Autodesk Fusion 360 part; units mm, degrees
sketch "Sketch1" plane through (0, 0, 0) normal (0, 0, 1) x (1, 0, 0)
  line L0 (89, 44) -> (69, 44)
  line L1 (43, -56) -> (63, -56)
  line L2 (-89, 24) -> (-69, 24)
  line L3 (-124, 33) -> (-124, 53)
  line L4 (-95, 36) -> (-95, 56)
  line L5 (174, 69) -> (-174, 69)
  line L6 (-174, -69) -> (174, -69)
  line L7 (170, 37) -> (150, 37)
  line L8 (150, 37) -> (150, -2)
  line L9 (-183, 60) -> (-183, -60)
  line L10 (-124, 53) -> (-144, 53)
  line L11 (115, 56) -> (95, 56)
  line L12 (-150, 37) -> (-170, 37)
  line L13 (-170, 37) -> (-170, 17)
  line L14 (-89, 44) -> (-89, 24)
  line L15 (-62, -36) -> (-62, -23)
  line L16 (-115, 36) -> (-95, 36)
  line L17 (-69, 24) -> (-69, 44)
  line L18 (-69, 44) -> (-89, 44)
  line L19 (-62, -23) -> (-82, -23)
  line L20 (124, 14) -> (144, 14)
  line L21 (-144, 33) -> (-124, 33)
  circle A0 centre (173, -59) radius 2.6
  line L22 (-10, -30) -> (10, -30)
  line L23 (82, -30) -> (101, -30)
  line L24 (-43, -56) -> (-43, -36)
  line L25 (-63, -43) -> (-63, -56)
  line L26 (-82, -43) -> (-63, -43)
  circle A1 centre (-173, -59) radius 2.6
  line L27 (-144, 53) -> (-144, 33)
  line L28 (-10, -10) -> (-10, -30)
  line L29 (-150, 17) -> (-150, 37)
  line L30 (-115, 56) -> (-115, 36)
  line L31 (-63, -56) -> (-43, -56)
  line L32 (-170, 17) -> (-150, 17)
  line L33 (82, 3) -> (62, 3)
  line L34 (115, 17) -> (115, 56)
  line L35 (43, -30) -> (62, -30)
  line L36 (170, -2) -> (170, 37)
  line L37 (95, 56) -> (95, 17)
  line L38 (63, -43) -> (82, -43)
  line L39 (89, 5) -> (89, 44)
  circle A2 centre (0, -59) radius 2.6
  line L40 (183, -60) -> (183, 60)
  circle A3 centre (-173, 59) radius 2.6
  line L41 (43, -36) -> (43, -56)
  line L42 (62, 3) -> (62, -10)
  line L43 (69, 44) -> (69, 5)
  line L44 (10, -10) -> (-10, -10)
  line L45 (43, -10) -> (43, -30)
  line L46 (101, -30) -> (101, -10)
  line L47 (144, 53) -> (124, 53)
  line L48 (62, -10) -> (43, -10)
  line L49 (82, -43) -> (82, -30)
  line L50 (-95, 56) -> (-115, 56)
  line L51 (-82, -23) -> (-82, -43)
  line L52 (124, 53) -> (124, 14)
  line L53 (150, -2) -> (170, -2)
  circle A4 centre (173, 59) radius 2.6
  line L54 (62, -30) -> (62, -36)
  line L55 (10, -30) -> (10, -10)
  line L56 (95, 17) -> (115, 17)
  line L57 (101, -10) -> (82, -10)
  line L58 (62, -36) -> (43, -36)
  line L59 (82, -10) -> (82, 3)
  line L60 (63, -56) -> (63, -43)
  line L61 (69, 5) -> (89, 5)
  line L62 (144, 14) -> (144, 53)
  line L63 (-43, -36) -> (-62, -36)
  arc A5 (-174, 69) -> (-183, 60) centre (-174, 60) ccw
  arc A6 (183, 60) -> (174, 69) centre (174, 60) ccw
  arc A7 (174, -69) -> (183, -60) centre (174, -60) ccw
  arc A8 (-183, -60) -> (-174, -69) centre (-174, -60) ccw
  circle A9 centre (33, 54) radius 3.5
  circle A10 centre (-33, 54) radius 3.5
  circle A11 centre (33, 20) radius 3.5
  circle A12 centre (-33, 20) radius 3.5
  circle A13 centre (53, 59) radius 2.6
  circle A14 centre (-53, 59) radius 2.6
  dimension "d1" = 9
  dimension "d2" = 7
  dimension "d3" = 7
  dimension "d4" = 7
  dimension "d5" = 7
  dimension "d8" = 5.2
  dimension "d9" = 5.2
extrude "Extrude1" add sketch "Sketch1" along normal blind 6
Input: part model. Units: mm. Frame: model coordinates. A direction names the side the tool comes from. Coordinates: 2 decimals unless noted, no trailing zeros. Loops run counter-clockwise (first coordinate to the right, second up) from the corner with the lowest first, then second, coordinate; pieces in that order, holes last. Notation, with made-up numbers: M 68.25,59.25 L 81.25,59.25 A29 cw 81.25,89.25 Z; hole C 84,65.25 d5. An arc over 180 degrees is marked long. Use a Markdown table: item, result. Add a question column.
1) Section C-C, the plane x = -159. Return the cut outline in (y, z), plus the area to 3 significant figures.
2) Draft query along X for faces 3 (the flat face through (183, -1, 3)), 4 (the flat face through (134, 53, 3)), 5 (the flat face through (-2, -69, 3)), 6 (the cylindrical face through (-33.46, 16.53, 2.96)). Return one class per face: +X half, -X half, draft (parallel to the pull), parting line (faces both ways), or undercut.
3) Section D-D, the plane z = 2.05. Give the number of separate pieces and of enclosed holes in the cut face, plus the area to 3 significant figures.
4) Line query: L1, parallel to X at y = -32.5, z = 0.85; L2, parallel to Y at x = 69.5, z = 1.25; L3, parallel to X at y = -19, z = 5.6. Output: solid intervals per line, ascending. Write a range as from..to.
5) Section A-A, the plane x = -33. Return the cut outline in (y, z), plus the area to 3 significant figures.
6) Section B-B, the plane y = -16. Return the cut outline in (x, z), plus the area to 3 significant figures.
7) Set-up query: faces 1 (the flat face through (69, 25, 3)), 2 (the flat face through (-3, 1, 0)). Return all of +Z, -Z, +X, -X, +Y, -Y with unobstructed straight access to the full face (end or side cutting, diameter ignored); none if empty.
Answer below:
| question | item | result |
|---|---|---|
| 1 | outline | M -69,0 L 17,0 L 17,6 L -69,6 Z; M 37,0 L 69,0 L 69,6 L 37,6 Z |
| 1 | area | 708 mm2 |
| 2 | face 3 | +X half |
| 2 | face 4 | undercut |
| 2 | face 5 | draft |
| 2 | face 6 | undercut |
| 3 | separate pieces | 1 |
| 3 | enclosed holes | 22 |
| 3 | area | 42,100 mm2 |
| 4 | L1 | -183..-82, -62..62, 82..183 |
| 4 | L2 | -69..-43, 3..5, 44..69 |
| 4 | L3 | -183..-10, 10..43, 101..183 |
| 5 | outline | M -69,0 L 16.5,0 L 16.5,6 L -69,6 Z; M 23.5,0 L 50.5,0 L 50.5,6 L 23.5,6 Z; M 57.5,0 L 69,0 L 69,6 L 57.5,6 Z |
| 5 | area | 744 mm2 |
| 6 | outline | M -183,0 L -10,0 L -10,6 L -183,6 Z; M 10,0 L 43,0 L 43,6 L 10,6 Z; M 101,0 L 183,0 L 183,6 L 101,6 Z |
| 6 | area | 1,730 mm2 |
| 7 | face 1 | +Z, -Z |
| 7 | face 2 | -Z, +X, -X, +Y, -Y |
